Part print with two shaded views. Sizes in mm from the minimum x, y, z corner. Round coordinates to 2 decimals unless told otherwise and drop trailing zeros. Order: outer loops, then holes, each group sorted by start corner. A loop starts at its lowest first (then second) coordinate and runs counter-clockwise, first axis right, second up. Notation, with made-up numbers: M 62.25,-26.5 L 114.25,-26.5 A25 cw 114.25,-4.5 Z; hole C -2.75,20 d3. An arc over 180 degrees is marked long. Answer as a JSON object with one key per item and string values.
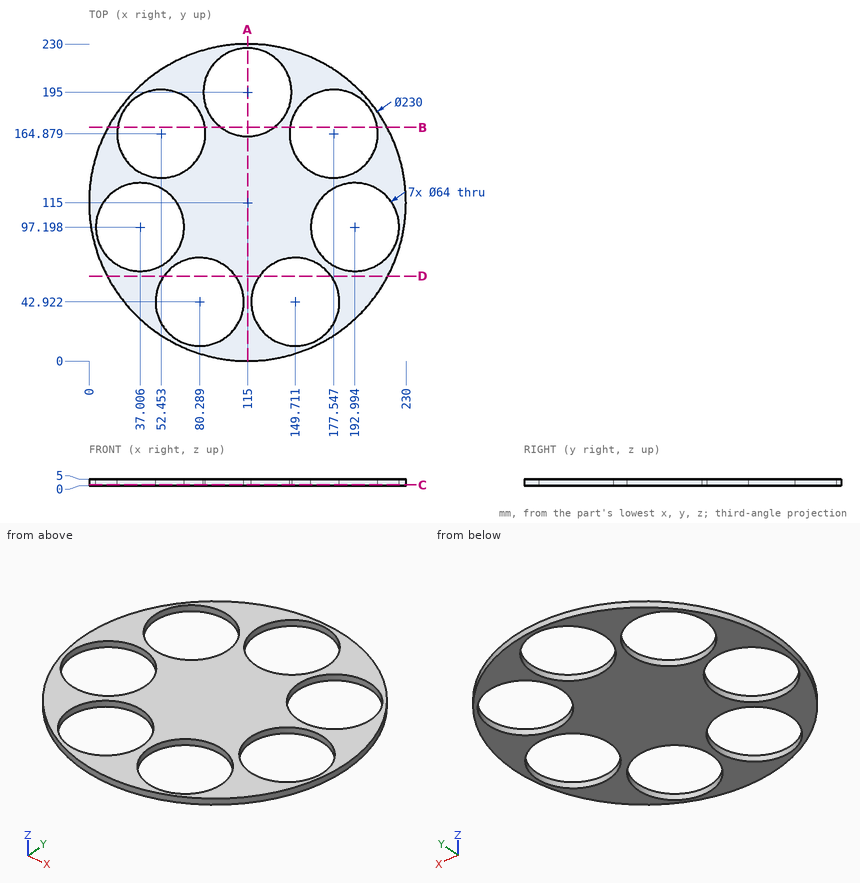
Item 1: Saw through at C-C on z = 0.75. List the corners of the cut face in (x, y) (1 decimal).
Worked answers:
{"outline": "C 115,115 d230; hole C 37,97.2 d64; hole C 52.5,164.9 d64; hole C 80.3,42.9 d64; hole C 115,195 d64; hole C 149.7,42.9 d64; hole C 177.5,164.9 d64; hole C 193,97.2 d64"}
Item 2: Saw through at D-D on y = 61.5. List the corners of the cut face in (x, z) (1 decimal), and give its area (3 significant figures).
Worked answers:
{"outline": "M 13.2,0 L 54.2,0 L 54.2,5 L 13.2,5 Z; M 106.3,0 L 123.7,0 L 123.7,5 L 106.3,5 Z; M 175.8,0 L 216.8,0 L 216.8,5 L 175.8,5 Z", "area": "497 mm2"}
Item 3: Saw through at B-B on y = 169.5. List the corners of the cut face in (x, z) (1 decimal), and give its area (3 significant figures).
Worked answers:
{"outline": "M 13.7,0 L 20.8,0 L 20.8,5 L 13.7,5 Z; M 84.1,0 L 95.7,0 L 95.7,5 L 84.1,5 Z; M 134.3,0 L 145.9,0 L 145.9,5 L 134.3,5 Z; M 209.2,0 L 216.3,0 L 216.3,5 L 209.2,5 Z", "area": "186 mm2"}
Item 4: Drop flat-ended pins along their axis: pin 1 Ø1.5 at (x, z) = (167.5, 2) entering from +Y; pin 2 Ø1 at (y, z) = (57, 2.5) entering from +X. Give the stop position or say it passes through.
Worked answers:
{"pin 1": "stops at y = 217.7", "pin 2": "stops at x = 214.59"}
Item 5: Saw through at A-A on x = 115. List the corners of the cut face in (y, z).
Worked answers:
{"outline": "M 0,0 L 163,0 L 163,5 L 0,5 Z; M 227,0 L 230,0 L 230,5 L 227,5 Z"}
Item 6: Wall check: line 1 along X through (y, z) = (158.5, 1.35) (1 decimal); line 2 along Y through (x, z) = (70.5, 2.8) (1 decimal); line 3 along Y through (x, z) = (115, 1.15). Give the ranges that are in metal, low to high. Write a range as [from, to].
Worked answers:
{"line 1": "x = [8.5, 21.1], [83.8, 146.2], [208.9, 221.5]", "line 2": "y = [9, 12.5], [73.4, 138.5], [191.3, 221]", "line 3": "y = [0, 163], [227, 230]"}
